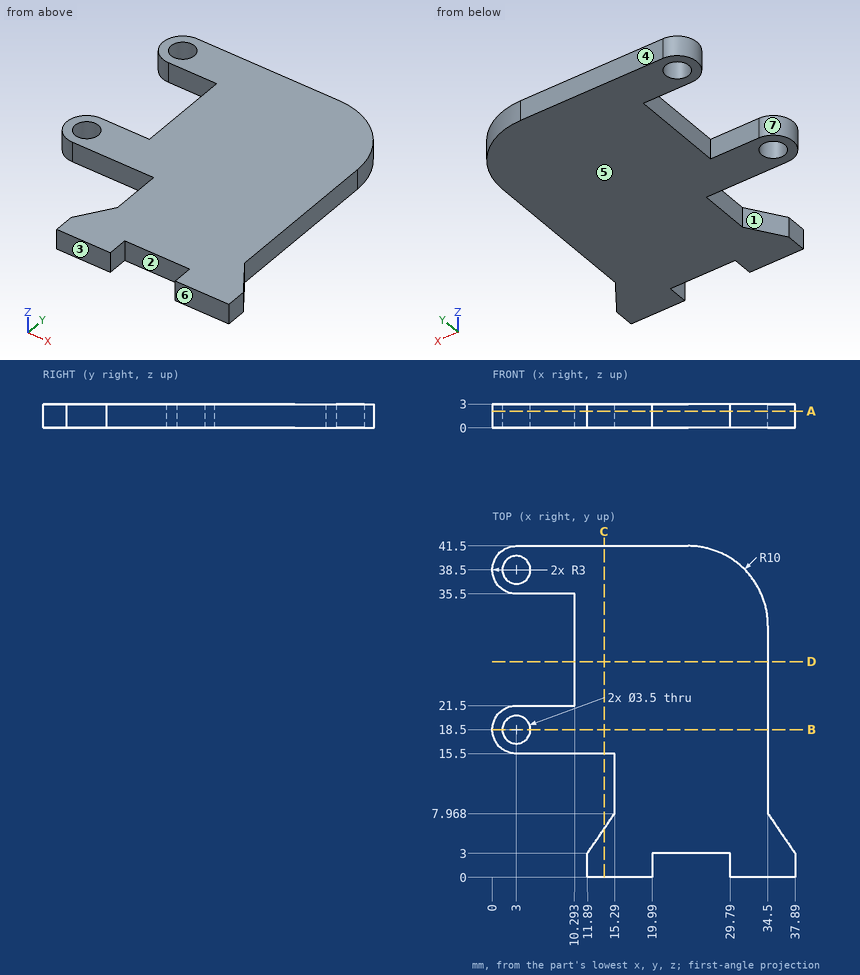
Study the drawing (mm; zero at the part's minimum x, y, z) and answer. A direction names the side the tool comes from. Give positions to 0.01 mm unless a question says otherwise; leave off trailing zeros. Order: outer loops, then holes, each group sorted by start corner. A loop starts at its lowest first (then second) coordinate and runs counter-clockwise, first axis right, second up. Notation, with made-up numbers: (76, 61.5) -> (118, 61.5) arc R15 cw to (118, 69.5) -> close; hole circle Ø5 at (37, 12). An arc over 180 degrees is marked (long way). Put each result on its own line as item: value.
Item 1: A cutting plane is placed at D-D on y = 27. Give the vertices of the cut face in (x, z).
Established:
outline: (10.29, 0) -> (34.5, 0) -> (34.5, 3) -> (10.29, 3) -> close
Item 2: For the marked faces 1, 2 and 3, determine the directions among +Z, -Z, +X, -X, +Y, -Y from which every point of the face is accessible in a straight line to the end or side of a thin tool.
Established:
face 1: +Z, -Z, -X
face 2: +Z, -Z, -Y
face 3: +Z, -Z, +X, -X, -Y
Item 3: A cutting plane is placed at A-A on z = 2.1. Give the vertices of the cut face in (x, y).
Established:
outline: (3, 15.5) -> (15.29, 15.5) -> (15.29, 7.97) -> (11.89, 3) -> (11.89, 0) -> (19.99, 0) -> (19.99, 3) -> (29.79, 3) -> (29.79, 0) -> (37.89, 0) -> (37.89, 3) -> (34.5, 7.97) -> (34.5, 31.5) arc R10 ccw to (24.5, 41.5) -> (3, 41.5) arc R3 ccw to (3, 35.5) -> (10.29, 35.5) -> (10.29, 21.5) -> (3, 21.5) arc R3 ccw to start; hole circle Ø3.5 at (3, 18.5); hole circle Ø3.5 at (3, 38.5)
Item 4: A cutting plane is placed at C-C on x = 14. Give the vertices of the cut face in (y, z).
Established:
outline: (0, 0) -> (6.08, 0) -> (6.08, 3) -> (0, 3) -> close; (15.5, 0) -> (41.5, 0) -> (41.5, 3) -> (15.5, 3) -> close
Item 5: For a pull along Y with two mould halves and no side action, classify the marked faces 4, 5, 6 and 7 as released by +Y, released by -Y, zero draft, split by the parting line, or undercut.
Established:
face 4: released by +Y
face 5: zero draft
face 6: released by -Y
face 7: undercut
Item 6: Straight lines are drawn through the part: line 1 (Y direction, x = 3, z = 1.4); line 2 (Y direction, x = 2, z = 2.75) (1 decimal); line 3 (X direction, y = 24, z = 2.5). For each, find the intervals that lie inside material, in ascending order.
Established:
line 1: y = 15.5 to 16.75, 20.25 to 21.5, 35.5 to 36.75, 40.25 to 41.5
line 2: y = 15.7 to 17.1, 19.9 to 21.3, 35.7 to 37.1, 39.9 to 41.3
line 3: x = 10.29 to 34.5
Item 7: A cutting plane is placed at B-B on y = 18.5. Give the vertices of the cut face in (x, z).
Established:
outline: (0, 0) -> (1.25, 0) -> (1.25, 3) -> (0, 3) -> close; (4.75, 0) -> (34.5, 0) -> (34.5, 3) -> (4.75, 3) -> close
Item 8: Given P1, Ø0.9, axis at y = 12.5, z = 2, coming from the -X side; P2, Ø0.9, axis at y = 18.5, z = 1, coming from the +X side; P3, Ø1, axis at x = 31.5, z = 2.5, coming from the +Y side, each flat-ended and moving along its own axis, determine where each tip first touches the part or whether it passes through.
Established:
P1: stops at x = 15.29
P2: stops at x = 34.5
P3: stops at y = 39.1
